```python
from build123d import *

# Parameters (mm, degrees)
SKETCH2_R                             = 50
BOSS_EXTRUDE2_DEPTH                   = 4
TAP_DRILL_FOR_M3X0_5_TAP1_D           = 2.5
TAP_DRILL_FOR_M3X0_5_TAP1_CSINK_D     = 2.55
TAP_DRILL_FOR_M3X0_5_TAP1_CSINK_ANGLE = 90
SKETCH5_W                             = 7
SKETCH5_H                             = 20.7
CUT_EXTRUDE1_DEPTH                    = 10


with BuildPart() as part:
    # Sketch2 → Boss-Extrude2 (new body)
    with BuildSketch(Plane(origin=(0, 0, 0), x_dir=(1, 0, 0), z_dir=(0, 1, 0))):
        Circle(SKETCH2_R)
    extrude(amount=BOSS_EXTRUDE2_DEPTH)

    # Tap Drill for M3x0.5 Tap1 (through all)
    with Locations(Plane(origin=(0, 4, 0), x_dir=(1, 0, 0), z_dir=(0, 1, 0))):
        with Locations((0, 6), (0, -6)):
            CounterSinkHole(TAP_DRILL_FOR_M3X0_5_TAP1_D / 2, TAP_DRILL_FOR_M3X0_5_TAP1_CSINK_D / 2, counter_sink_angle=TAP_DRILL_FOR_M3X0_5_TAP1_CSINK_ANGLE)

    # Sketch5 → Cut-Extrude1 (cut)
    with BuildSketch(Plane.XZ):
        with Locations((-42.5, 0)):
            Rectangle(SKETCH5_W, SKETCH5_H)
        with Locations((42.5, 0)):
            Rectangle(SKETCH5_W, SKETCH5_H)
    extrude(amount=-CUT_EXTRUDE1_DEPTH, mode=Mode.SUBTRACT)


solid = part.part
```
Verification items for the finished model (mm, model axes). A direction names the side the tool comes from. Round coordinates to 2 decimals unless told otherwise and drop trailing zeros. Loops run counter-clockwise (first coordinate to the right, second up) from the corner with the lowest first, then second, coordinate; pieces in that order, holes last. Notation, with made-up numbers: (61, 17) -> (82, 17) arc R23 cw to (82, 46) -> close; hole circle Ø6 at (-18.5, 28). An arc over 180 degrees is marked (long way). Answer as a JSON object with one key per item and string values.
Q1. Section check C-C (y = 1.45). Record the boundary of the cut face in (x, z).
Data:
{"outline": "circle Ø100 at (0, 0); hole (-46, -10.35) -> (-39, -10.35) -> (-39, 10.35) -> (-46, 10.35) -> close; hole circle Ø2.5 at (0, -6); hole circle Ø2.5 at (0, 6); hole (39, -10.35) -> (46, -10.35) -> (46, 10.35) -> (39, 10.35) -> close"}
Q2. Section check A-A (z = 0). Record the boundary of the cut face in (x, y), then the cut area to 3 significant figures.
Data:
{"outline": "(-50, 0) -> (-46, 0) -> (-46, 4) -> (-50, 4) -> close; (-39, 0) -> (39, 0) -> (39, 4) -> (-39, 4) -> close; (46, 0) -> (50, 0) -> (50, 4) -> (46, 4) -> close", "area": "344 mm2"}
Q3. Scan lines: line 1 (Z direction, x = 0, y = 2.05); line 2 (X direction, y = 1.75, z = 6); line 3 (Z direction, x = -1, y = 1.75). Record each from-to range of solid material in increasing order. Write a range as from..to.
Data:
{"line 1": "z = -50..-7.25, -4.75..4.75, 7.25..50", "line 2": "x = -49.64..-46, -39..-1.25, 1.25..39, 46..49.64", "line 3": "z = -49.99..-6.75, -5.25..5.25, 6.75..49.99"}
Q4. Section check B-B (x = 0). Record the boundary of the cut face in (y, z) (3 decimals).
Data:
{"outline": "(0, -50) -> (4, -50) -> (4, -7.275) -> (3.975, -7.25) -> (0, -7.25) -> close; (0, -4.75) -> (3.975, -4.75) -> (4, -4.725) -> (4, 4.725) -> (3.975, 4.75) -> (0, 4.75) -> close; (0, 7.25) -> (3.975, 7.25) -> (4, 7.275) -> (4, 50) -> (0, 50) -> close"}
Q5. Draft check along Z on faces 1 (the flat face through (42, 2, -10.35)), 2 (the flat face through (-1, 0, -1)), 3 (the cylindrical face through (47.69, 1.97, -15.02)). Enter one of: pulls with the +Z half, pulls with the -Z half, needs draft (parallel to the pull), parting line crosses it, or undercut.
Data:
{"face 1": "undercut", "face 2": "needs draft", "face 3": "parting line crosses it"}
Q6. Section check D-D (x = 36.5). Record the boundary of the cut face in (y, z).
Data:
{"outline": "(0, -34.17) -> (4, -34.17) -> (4, 34.17) -> (0, 34.17) -> close"}
Q7. Go/stop test with flat-tipped pins: P1, Ø1.2, axis at y = 2.5, z = -4, coming from the +X side; P2, Ø1.2, axis at x = -44, y = 2.5, coming from the -Z side; P3, Ø2, axis at y = 2.5, z = 6.5, coming from the -X side; P4, Ø1.5, axis at x = 0, z = -6, coming from the -Y side. Record where each tip stops, or that it passes through.
Data:
{"P1": "stops at x = 49.88", "P2": "stops at z = -24.83", "P3": "stops at x = -49.7", "P4": "passes through"}
Q8. Access from +Z, -Z, +X, -X, +Y, -Y to the whole of each face (thin tool, end or side, straight path). Record for faces 4 (the flat face through (-1, 4, -1)), 5 (the flat face through (-43, 2, 10.35)).
Data:
{"face 4": "+Z, -Z, +X, -X, +Y", "face 5": "+Y, -Y"}
